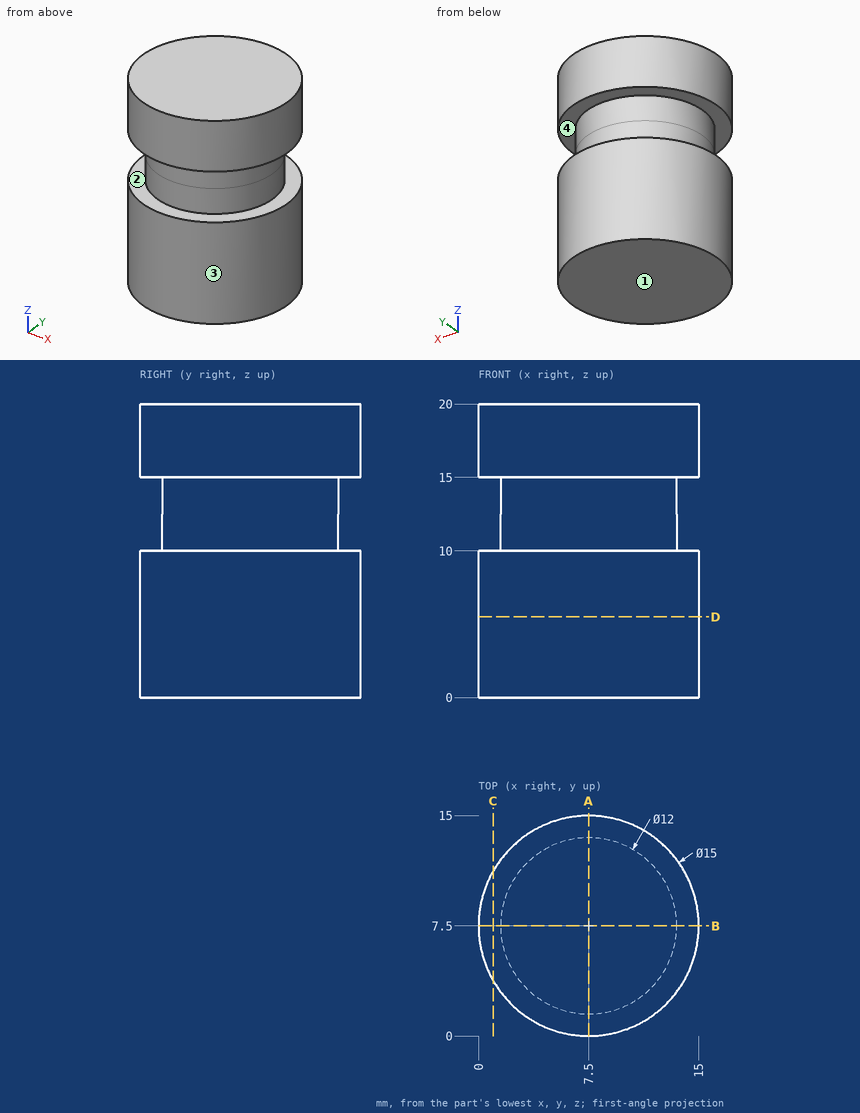
Check sheet for the drawn part. Datum: minimum x, y, z corner. Units: mm. Round coordinates to 2 decimals unless told otherwise and drop trailing zeros. Loops run counter-clockwise (first coordinate to the right, second up) from the corner with the lowest first, then second, coordinate; pieces in that order, holes last. Notation, with made-up numbers: M 56.25,60.5 L 99.25,60.5 A18 cw 99.25,65.5 Z; hole C 46.5,38 d1. An arc over 180 degrees is marked long. One line per question, with ' | ' between items. Start each with the question number.
Item 1: Scan lines: probe 1 along Z at (x, y) = (2, 11); probe 2 along Y at (x, z) = (12, 15.75); probe 3 along Y at (x, z) = (7.25, 6). Record each from-to range of solid material in increasing order.
Item 2: Section check A-A (x = 7.5). Record the boundary of the cut face in (y, z), and give its area (3 significant figures).
Item 3: Section check C-C (x = 1). Record the boundary of the cut face in (y, z), and give its area (3 significant figures).
Item 4: Release check for a two-part mould opening along Z. For the marked faces 1, 2, 3 and 4 record: released by +Z, released by -Z, zero draft, split by the parting line, or undercut.
Item 5: Section check D-D (z = 5.5). Record the boundary of the cut face in (x, y), and give its area (3 significant figures).
Item 6: Gauge pin test, flat ends, axial feed: pin 1 Ø1.5 at (y, z) = (13, 6.5) entering from +X; pin 2 Ø3 at (y, z) = (5.5, 16.5) entering from +X. Record the tip position at first contact, or that the pin passes through.
Worked out:
1) probe 1: 0 to 10, 15 to 20 | probe 2: 1.5 to 13.5 | probe 3: 0 to 15
2) outline: M 0,0 L 15,0 L 15,10 L 13.5,10 L 13.5,15 L 15,15 L 15,20 L 0,20 L 0,15 L 1.5,15 L 1.5,10 L 0,10 Z | area: 285 mm^2
3) outline: M 3.76,0 L 11.24,0 L 11.24,10 L 3.76,10 Z; M 3.76,15 L 11.24,15 L 11.24,20 L 3.76,20 Z | area: 112 mm^2
4) face 1: released by -Z | face 2: undercut | face 3: zero draft | face 4: undercut
5) outline: C 7.5,7.5 d15 | area: 177 mm^2
6) pin 1: x = 13.3 | pin 2: x = 14.98
